```python
from build123d import *

# Parameters (mm, degrees)
SKETCH_1_R                      = 1.6
SKETCH_1_W                      = 105
SKETCH_1_H                      = 48
EXTRUDE_1_DEPTH                 = 2
FILLET_1_R                      = 3
SKETCH_2_W                      = 30
SKETCH_2_H                      = 2
EXTRUDE_2_DEPTH                 = 32
CUT_EXTRUDE_START               = -2
CUT_EXTRUDE_1_OUTLINE_R         = 6
CUT_EXTRUDE_1_DEPTH             = 2
SKETCH_4_W                      = 42
SKETCH_4_H                      = 2
EXTRUDE_3_DEPTH                 = 44
CUT_EXTRUDE_2_REACH             = 144.849
SKETCH_5_R                      = 2.1
SKETCH_5_R_2                    = 12.5
CUT_EXTRUDE_2_DIRECTION_2_DEPTH = 143.84882365


# Read off the part's stored shape, not the designer's step: ｶｯﾄ - 押し出し1
with BuildPart() as part:
    # ｽｹｯﾁ1 → ﾎﾞｽ - 押し出し1 (new body)
    with BuildSketch(Plane.XY):
        with BuildLine():
            Line((-116.941733701, 29), (116.941733701, 29))
            ThreePointArc((116.941733701, 29), (121.697016283, 25.545084972), (119.880659963, 19.954915028))
            Line((119.880659963, 19.954915028), (52.5, -29))
            Line((52.5, -29), (-52.5, -29))
            Line((-52.5, -29), (-119.880659963, 19.954915028))
            ThreePointArc((-119.880659963, 19.954915028), (-121.697016283, 25.545084972), (-116.941733701, 29))
        make_face()
        with Locations((118.411196832, 21.977457514)):
            Circle(SKETCH_1_R, mode=Mode.SUBTRACT)
        with Locations((77.960347113, -7.411805101)):
            Circle(SKETCH_1_R, mode=Mode.SUBTRACT)
        with Locations(Location((-118.411196832, 21.977457514, 0), (0, 0, 180))):
            Circle(SKETCH_1_R, mode=Mode.SUBTRACT)
        with Locations(Location((-77.960347113, -7.411805101, 0), (0, 0, 180))):
            Circle(SKETCH_1_R, mode=Mode.SUBTRACT)
        Rectangle(SKETCH_1_W, SKETCH_1_H, mode=Mode.SUBTRACT)
        with BuildLine():
            Line((-57.5, 21), (-57.5, -13.299115956))
            ThreePointArc((-57.5, -13.299115956), (-59.138028501, -15.972135529), (-62.263355757, -15.726166939))
            Line((-62.263355757, -15.726166939), (-116.941733701, 24))
            Line((-116.941733701, 24), (-60.5, 24))
            ThreePointArc((-60.5, 24), (-58.378679656, 23.121320344), (-57.5, 21))
        make_face(mode=Mode.SUBTRACT)
        with BuildLine():
            Line((62.263355757, -15.726166939), (116.941733701, 24))
            Line((116.941733701, 24), (60.5, 24))
            ThreePointArc((60.5, 24), (58.378679656, 23.121320344), (57.5, 21))
            Line((57.5, 21), (57.5, -13.299115956))
            ThreePointArc((57.5, -13.299115956), (59.138028501, -15.972135529), (62.263355757, -15.726166939))
        make_face(mode=Mode.SUBTRACT)
    extrude(amount=EXTRUDE_1_DEPTH)

    # ﾌｨﾚｯﾄ1
    fillet_1_edges = [part.edges().sort_by_distance(p)[0] for p in [
        (-52.5, -29, 1),
        (-52.5, 24, 1),
        (-52.5, -24, 1),
        (52.5, -24, 1),
        (52.5, 24, 1),
        (116.941733701, 24, 1),
        (-116.941733701, 24, 1),
    ]]
    fillet(fillet_1_edges, radius=FILLET_1_R)

    # ｽｹｯﾁ2 → ﾎﾞｽ - 押し出し2 (add)
    with BuildSketch(Plane(origin=(0, 0, 0), x_dir=(-1, 0, 0), z_dir=(0, 0, -1))):
        with Locations((-0.436960971, -23)):
            Rectangle(SKETCH_2_W, SKETCH_2_H)
    extrude(amount=-EXTRUDE_2_DEPTH)

    # ｶｯﾄ - 押し出し1 outline → ｶｯﾄ - 押し出し1 (cut)
    with BuildSketch(Plane.XZ.offset(24).offset(CUT_EXTRUDE_START)):
        with BuildLine():
            ThreePointArc((-14.563039029, 17), (-10.169640747, 27.606601718), (0.436960971, 32))
            Line((0.436960971, 32), (-14.563039029, 32))
            Line((-14.563039029, 32), (-14.563039029, 17))
        make_face()
        with BuildLine():
            ThreePointArc((0.436960971, 32), (11.043562689, 27.606601718), (15.436960971, 17))
            Line((15.436960971, 17), (15.436960971, 32))
            Line((15.436960971, 32), (0.436960971, 32))
        make_face()
        with Locations((0.436960971, 23)):
            Circle(CUT_EXTRUDE_1_OUTLINE_R)
    extrude(amount=CUT_EXTRUDE_1_DEPTH, mode=Mode.SUBTRACT)

    # ｽｹｯﾁ4 → ﾎﾞｽ - 押し出し3 (add)
    with BuildSketch(Plane(origin=(0, 0, 0), x_dir=(-1, 0, 0), z_dir=(0, 0, -1))):
        with Locations((0, 30)):
            Rectangle(SKETCH_4_W, SKETCH_4_H)
    extrude(amount=-EXTRUDE_3_DEPTH)

    # ｽｹｯﾁ5 → ｶｯﾄ - 押し出し2 (cut, up to next)
    with BuildSketch(Plane(origin=(0, 31, 0), x_dir=(1, 0, 0), z_dir=(0, 1, 0)), mode=Mode.PRIVATE) as cut_extrude_2_sk1:
        with Locations(Location((0, -5.5, 0), (0, 0, 90))):
            Circle(SKETCH_5_R)
    cut_extrude_2_tool1 = extrude(cut_extrude_2_sk1.sketch, amount=-CUT_EXTRUDE_2_REACH, mode=Mode.PRIVATE) & part.part
    # ｽｹｯﾁ5 → ｶｯﾄ - 押し出し2 (cut, up to next)
    with BuildSketch(Plane(origin=(0, 31, 0), x_dir=(1, 0, 0), z_dir=(0, 1, 0)), mode=Mode.PRIVATE) as cut_extrude_2_sk2:
        with Locations(Location((-17.5, -23, 0), (0, 0, 90))):
            Circle(SKETCH_5_R)
    cut_extrude_2_tool2 = extrude(cut_extrude_2_sk2.sketch, amount=-CUT_EXTRUDE_2_REACH, mode=Mode.PRIVATE) & part.part
    # ｽｹｯﾁ5 → ｶｯﾄ - 押し出し2 (cut, up to next)
    with BuildSketch(Plane(origin=(0, 31, 0), x_dir=(1, 0, 0), z_dir=(0, 1, 0)), mode=Mode.PRIVATE) as cut_extrude_2_sk3:
        with Locations(Location((0, -40.5, 0), (0, 0, 90))):
            Circle(SKETCH_5_R)
    cut_extrude_2_tool3 = extrude(cut_extrude_2_sk3.sketch, amount=-CUT_EXTRUDE_2_REACH, mode=Mode.PRIVATE) & part.part
    # ｽｹｯﾁ5 → ｶｯﾄ - 押し出し2 (cut, up to next)
    with BuildSketch(Plane(origin=(0, 31, 0), x_dir=(1, 0, 0), z_dir=(0, 1, 0)), mode=Mode.PRIVATE) as cut_extrude_2_sk4:
        with Locations(Location((17.5, -23, 0), (0, 0, 90))):
            Circle(SKETCH_5_R)
    cut_extrude_2_tool4 = extrude(cut_extrude_2_sk4.sketch, amount=-CUT_EXTRUDE_2_REACH, mode=Mode.PRIVATE) & part.part
    # ｽｹｯﾁ5 → ｶｯﾄ - 押し出し2 (cut, up to next)
    with BuildSketch(Plane(origin=(0, 31, 0), x_dir=(1, 0, 0), z_dir=(0, 1, 0)), mode=Mode.PRIVATE) as cut_extrude_2_sk5:
        with Locations(Location((0, -23, 0), (0, 0, 90))):
            Circle(SKETCH_5_R_2)
    cut_extrude_2_tool5 = extrude(cut_extrude_2_sk5.sketch, amount=-CUT_EXTRUDE_2_REACH, mode=Mode.PRIVATE) & part.part
    add(cut_extrude_2_tool1.solids().sort_by_distance((0, 31, 5.5))[0], mode=Mode.SUBTRACT)
    add(cut_extrude_2_tool2.solids().sort_by_distance((-17.5, 31, 23))[0], mode=Mode.SUBTRACT)
    add(cut_extrude_2_tool3.solids().sort_by_distance((0, 31, 40.5))[0], mode=Mode.SUBTRACT)
    add(cut_extrude_2_tool4.solids().sort_by_distance((17.5, 31, 23))[0], mode=Mode.SUBTRACT)
    add(cut_extrude_2_tool5.solids().sort_by_distance((0, 31, 23))[0], mode=Mode.SUBTRACT)

    # ｽｹｯﾁ5 → ｶｯﾄ - 押し出し2 direction 2 (cut)
    with BuildSketch(Plane(origin=(0, 31, 0), x_dir=(1, 0, 0), z_dir=(0, 1, 0))):
        with Locations(Location((0, -5.5, 0), (0, 0, 90))):
            Circle(SKETCH_5_R)
        with Locations(Location((-17.5, -23, 0), (0, 0, 90))):
            Circle(SKETCH_5_R)
        with Locations(Location((0, -40.5, 0), (0, 0, 90))):
            Circle(SKETCH_5_R)
        with Locations(Location((17.5, -23, 0), (0, 0, 90))):
            Circle(SKETCH_5_R)
        with Locations(Location((0, -23, 0), (0, 0, 90))):
            Circle(SKETCH_5_R_2)
    extrude(amount=CUT_EXTRUDE_2_DIRECTION_2_DEPTH, mode=Mode.SUBTRACT)


solid = part.part
```
The listing builds one solid part. Answer for the finished solid, in the listing's coordinates (mm). A direction names the side the tool comes from. Give positions to 0.01 mm unless a question says otherwise; leave off trailing zeros. Write each loop counter-clockwise with the first axis right and the second up, starting at its lowest first coordinate (ties: lowest second). Pieces come first, ordered by that corner, then holes. Notation, with made-up numbers: (49.25, -5) - (73.25, -5) arc R27 cw to (73.25, 21) - close; hole circle Ø9 at (52.5, 40). An arc over 180 degrees is marked (long way). Use one line per item in the form item = value. Start each with the question number.
1) Find section A-A on z = 40.5. Determine the outline of the cut face in (x, y).
2) Find section C-C on z = 5.5. Determine the outline of the cut face in (x, y).
3) The mould has two halves that part along Z. Classify faces 1 (the face through (15.418, 30.014, 23.273)), 2 (the face through (10, 29, 13)), 3 (the face through (1, 28, 0)): pulls with the +Z half, pulls with the -Z half, needs draft (parallel to the pull), parting line crosses it, or undercut.
4) Consider line 1 along X through (y, z) = (30, 23); line 2 along Z through (x, y) = (-17.5, 30.05); line 3 along Y through (x, z) = (-4.5, 28.5). Determine where each line is inside the solid, lowest interval first. Write a range as from..to.
5) A tool of negligible diameter and unlimited length cuts with its end or side. For faces 4 (the face through (-85.537, 1.183, 0.986)), 5 (the face through (-0.09, 30.01, 42.6)), 6 (the face through (-8.45, 30.01, 32.21)), 7 (the face through (1, -24, 13)), from which of +Z, -Z, +X, -X, +Y, -Y can it reach the whole face along a straight path? Write none if from no direction.
6) Flat-ended cylindrical pins translate along their axes: pin 1 Ø1.6 at (x, z) = (-68.5, 1) entering from +Y; pin 2 Ø3 at (x, z) = (-9, 31) entering from -Y; pin 3 Ø0.6 at (y, z) = (29.5, 23) entering from +X; pin 4 Ø3 at (x, y) = (118.41, 21.98) entering from -Z. Find the tip coordinate at first contact, or state that the pin passes through.
7) Find section B-B on x = -17.5. Determine the outline of the cut face in (y, z).
8) Find section D-D on y = 15. Determine the outline of the cut face in (x, z), plus the area to 3 significant figures.
Geometry results:
q1.outline = (-21, 29) - (-2.1, 29) - (-2.1, 31) - (-21, 31) - close; (2.1, 29) - (21, 29) - (21, 31) - (2.1, 31) - close
q2.outline = (-21, 29) - (-2.1, 29) - (-2.1, 31) - (-21, 31) - close; (-14.56, -24) - (15.44, -24) - (15.44, -22) - (-14.56, -22) - close; (2.1, 29) - (21, 29) - (21, 31) - (2.1, 31) - close
q3.face_1 = undercut
q3.face_2 = needs draft
q3.face_3 = pulls with the -Z half
q4.line_1 = -21..-19.6, -15.4..-12.5, 12.5..15.4, 19.6..21
q4.line_2 = 0..20.9, 25.1..44
q4.line_3 = -24..-22
q5.face_4 = +Z, -Z
q5.face_5 = +Y, -Y
q5.face_6 = +Y
q5.face_7 = +Z, +X, -X, -Y
q6.pin_1 = 29
q6.pin_2 = 29
q6.pin_3 = 21
q6.pin_4 = through
q7.outline = (-29, 0) - (-24, 0) - (-24, 2) - (-29, 2) - close; (24, 0) - (31, 0) - (31, 20.9) - (29, 20.9) - (29, 2) - (24, 2) - close; (29, 25.1) - (31, 25.1) - (31, 44) - (29, 44) - close
q8.outline = (-113.06, 0) - (-104.55, 0) - (-104.55, 2) - (-113.06, 2) - close; (-57.5, 0) - (-52.5, 0) - (-52.5, 2) - (-57.5, 2) - close; (52.5, 0) - (57.5, 0) - (57.5, 2) - (52.5, 2) - close; (104.55, 0) - (113.06, 0) - (113.06, 2) - (104.55, 2) - close
q8.area = 54.0 mm2
